from build123d import *

# Parameters (mm, degrees)
SKETCH5_W          = 34
SKETCH5_H          = 34
CUT_EXTRUDE1_DEPTH = 3
SKETCH6_W          = 3
SKETCH6_H          = 11.7
SKETCH7_W          = 4.8
SKETCH7_H          = 1


with BuildPart() as part:
    # Sketch1 → Revolve1 (revolve)
    with BuildSketch(Plane.XY):
        Polygon((0, 34), (4.615384615, 34), (4.615384615, 33), (3.6, 33), (3.6, 32), (4, 32), (4, 12), (4.8, 12), (4.8, 9.5), (3.157894737, 9.5), (3.157894737, 8), (0, 8), align=None)
    revolve(axis=Axis((0, 8, 0), (0, 1, 0)))

    # Sketch2 → Revolve2 (revolve)
    with BuildSketch(Plane.XY):
        Polygon((0, 30.5), (5.3865, 30.5), (6, 29.8865), (6, 13.6135), (5.3865, 13), (0, 13), align=None)
    revolve(axis=Axis((0, 13, 0), (0, 1, 0)))

    # Sketch3 → Revolve3 (revolve)
    with BuildSketch(Plane.XY):
        Polygon((0, 32), (3.5, 32), (4, 31.3), (4.3, 31.3), (4.5, 31.1), (4.5, 30.5), (0, 30.5), align=None)
    revolve(axis=Axis((0, 30.5, 0), (0, 1, 0)))

    # Sketch4 → Revolve4 (revolve)
    with BuildSketch(Plane.XY):
        Polygon((0, 12), (6, 12), (7.2, 11.678460969), (7.2, 9), (8, 9), (8, 8), (0, 8), align=None)
    revolve(axis=Axis((0, 8, 0), (0, 1, 0)))

    # Sketch5 → Cut-Extrude1 (cut)
    with BuildSketch(Plane(origin=(0, 12, 0), x_dir=(-1, 0, 0), z_dir=(0, 1, 0))):
        Rectangle(SKETCH5_W, SKETCH5_H)
        Polygon((6.92820323, 0), (3.464101615, 6), (-3.464101615, 6), (-6.92820323, 0), (-3.464101615, -6), (3.464101615, -6), align=None, mode=Mode.SUBTRACT)
    extrude(amount=-CUT_EXTRUDE1_DEPTH, mode=Mode.SUBTRACT)

    # Sketch6 → Cut-Revolve1 (revolve, cut)
    with BuildSketch(Plane.XY):
        with Locations((1.5, 28.15)):
            Rectangle(SKETCH6_W, SKETCH6_H)
    revolve(axis=Axis((0, 22.3, 0), (0, 1, 0)), mode=Mode.SUBTRACT)

    # Sketch7 → Revolve5 (revolve)
    with BuildSketch(Plane.XY):
        with Locations((2.4, 12.5)):
            Rectangle(SKETCH7_W, SKETCH7_H)
    revolve(axis=Axis((0, 12, 0), (0, 1, 0)))


solid = part.part
Input: part model. Units: mm. Frame: model coordinates. A direction names the side the tool comes from. Round coordinates to 2 decimals unless told otherwise and drop trailing zeros. Order: outer loops, then holes, each group sorted by start corner. A loop starts at its lowest first (then second) coordinate and runs counter-clockwise, first axis right, second up. Notation, with made-up numbers: (-15.5, 33.25) - (42.5, 33.25) arc R21 cw to (42.5, 40.25) - close; hole circle Ø8 at (17, -38.5). An arc over 180 degrees is marked (long way). Answer as a JSON object with one key per item and string values. Group by question number.
(1) Reachability of faces 1 (the face through (0, 11, 6)), 2 (the face through (-0.59, 30.8, -4.46)), 3 (the face through (-1, 34, 3)), 4 (the face through (-3.66, 33.49, 2.81)), 5 (the face through (0, 8, 0)) from +Z, -Z, +X, -X, +Y, -Y: full face, straight path, thin tool, end or side. Return the list, or none.
(2) Cut plane B-B (y = 21). Return loops of the section in (x, z), then the cut area to 3 significant figures.
(3) Draft query along X for faces 6 (the face through (-4, 13, 3)), 7 (the face through (0, 22.3, 0)), 8 (the face through (2.58, 12.51, -4.05)). Return one class per face: released by +X, released by -X, zero draft, split by the parting line, or undercut.
(4) Cut plane A-A (y = 11.25). Return loops of the section in (x, z).
(5) Pin query (flat end, axial travel): P1, Ø2.5, axis at x = 0, y = 10.5, coming from the -Z side; P2, Ø5.5, axis at x = 0, z = 0, coming from the +Y side; P3, Ø9.5, axis at x = 0.5, z = 2, coming from the +Y side; P4, Ø5, axis at y = 25.5, z = 0.5, coming from the +X side. Return the tip coordinate at first contact, or that it passes through.
(6) Material intervals for probe 1 along Z at (x, y) = (0, 25); probe 2 along Y at (x, z) = (0.75, -4.5), sorted ascending. Write a range as from..to.
Here are the results:
{
 "1": {"face 1": "+Z, +X, -X, +Y", "face 2": "none", "face 3": "+Z, -Z, +X, -X, +Y", "face 4": "+Y", "face 5": "+Z, -Z, +X, -X, -Y"},
 "2": {"outline": "circle Ø12 at (0, 0)", "area": "113 mm^2"},
 "3": {"face 6": "zero draft", "face 7": "undercut", "face 8": "split by the parting line"},
 "4": {"outline": "(-6.93, 0) - (-3.46, -6) - (3.46, -6) - (6.93, 0) - (3.46, 6) - (-3.46, 6) - close"},
 "5": {"P1": "stops at z = -6", "P2": "stops at y = 22.3", "P3": "stops at y = 34", "P4": "stops at x = 6"},
 "6": {"probe 1": "z = -6..-3, 3..6", "probe 2": "y = 8..30.5, 33..34"}
}
